Model file for the job. Use its own axes, mm. Give positions to 0.01 mm unless a question says otherwise; leave off trailing zeros. Order: outer loops, then holes, each group sorted by start corner. A loop starts at its lowest first (then second) coordinate and runs counter-clockwise, first axis right, second up. Notation, with made-up numbers: M 3,2.25 L 31,2.25 A34 ccw 31,39.25 Z; hole C 27.5,20 d7. An arc over 180 degrees is marked long. Return JSON: item names as keys, results as strings. Group by question number.
1. Slice it at A-A on x = 6. List the corners of the cut face in (y, z), then the cut area to 3 significant figures.
2. Wall check: probe 1 along X at (y, z) = (16.75, 0.8); probe 2 along X at (y, z) = (17, 0.45); probe 3 along Y at (x, z) = (16.89, 0.5). Give the ranges that are in metal, low to high. Write a range as [from, to].
3. Two-plate mould, pull along X, no slides. Class faces 1 (the face through (2.283, 17.526, 0.789)), 2 (the face through (17.78, 9, 1)), 3 (the face through (0.752, 0.713, 0.789)): released by +X, released by -X, zero draft, split by the parting line, or undercut.
4. Slice it at C-C on x = 0.89. List the corners of the cut face in (y, z).
5. Slice it at B-B on z = 0.45. Give the number of separate pieces and of enclosed holes in the cut face, then the cut area to 3 significant figures.
Autodesk Fusion 360 part; units mm, degrees
sketch "Skizze1" plane through (0, 0, 0) normal (0, 0, 1) x (1, 0, 0)
  line L0 (2.5, 0) -> (15.28, 0)
  line L1 (17.78, 2.5) -> (17.78, 16.55)
  line L2 (15.28, 19.05) -> (2.5, 19.05)
  line L3 (0, 16.55) -> (0, 2.5)
  arc A0 (2.5, 19.05) -> (0, 16.55) centre (2.5, 16.55) ccw
  arc A1 (17.78, 16.55) -> (15.28, 19.05) centre (15.28, 16.55) ccw
  arc A2 (15.28, 0) -> (17.78, 2.5) centre (15.28, 2.5) ccw
  arc A3 (0, 2.5) -> (2.5, 0) centre (2.5, 2.5) ccw
  circle A4 centre (2.5, 16.55) radius 1
  circle A5 centre (15.2, 16.55) radius 1
  circle A6 centre (0.89, 2.5) radius 0.5
  circle A7 centre (3.5567, 2.5) radius 0.5
  circle A8 centre (6.2233, 2.5) radius 0.5
  circle A9 centre (8.89, 2.5) radius 0.5
  circle A10 centre (11.5567, 2.5) radius 0.5
  circle A11 centre (14.2233, 2.5) radius 0.5
  circle A12 centre (16.89, 2.5) radius 0.5
  point P0 (17.78, 0)
  dimension "d3" = 17.78
  dimension "d4" = 19.05
  dimension "d5" = 2.5
  dimension "d6" = 2
  dimension "d9" = 12.7
  dimension "d10" = 0
  dimension "d11" = 1
  dimension "d12" = 2.5
  dimension "d15" = 16
  dimension "d16" = 0
  dimension "d17" = 8.89
extrude "Extrusion1" add sketch "Skizze1" along normal blind 1.6
Result:
{
 "1": {"outline": "M 0,0 L 2.05,0 L 2.05,1.6 L 0,1.6 Z; M 2.95,0 L 19.05,0 L 19.05,1.6 L 2.95,1.6 Z", "area": "29.0 mm2"},
 "2": {"probe 1": "x = [0.01, 1.52], [3.48, 14.22], [16.18, 17.77]", "probe 2": "x = [0.04, 1.61], [3.39, 14.31], [16.09, 17.74]", "probe 3": "y = [0.59, 2], [3, 18.46]"},
 "3": {"face 1": "undercut", "face 2": "released by +X", "face 3": "released by -X"},
 "4": {"outline": "M 0.59,0 L 2,0 L 2,1.6 L 0.59,1.6 Z; M 3,0 L 18.46,0 L 18.46,1.6 L 3,1.6 Z"},
 "5": {"separate pieces": "1", "enclosed holes": "9", "area": "322 mm2"}
}
